```python
from build123d import *

# Parameters (mm, degrees)
F2_R        = 42.2275
F0_DEPTH    = 11.1125
F3_T        = -3.175
F0_FACE_R   = 42.2275
F0_FACE_R_2 = 39.0525
F4_DEPTH    = 25.4


with BuildPart() as f0:
    # F2 (on Top) → F0 (new body)
    with BuildSketch(Plane.XY):
        Circle(F2_R)
    extrude(amount=-F0_DEPTH)

    # F3
    f3_openings = [f0.faces().sort_by_distance(p)[0] for p in [
        (0, 0, 0),
    ]]
    offset(amount=F3_T, openings=f3_openings)

    # F1 (on face) + F0_face (on face) → F4 (cut)
    with BuildSketch(Plane.XY.offset(-7.9375)):
        with BuildLine():
            ThreePointArc((-18.689399569, -34.29), (-39.0525, 0), (-18.689399569, 34.29))
            Line((-18.689399569, 34.29), (-44.45, 34.29))
            Line((-44.45, 34.29), (-44.45, -34.29))
            Line((-44.45, -34.29), (-18.689399569, -34.29))
        make_face()
        with BuildLine():
            ThreePointArc((-5.9242471252, -34.29), (-34.798, 0), (-5.9242471252, 34.29))
            Line((-5.9242471252, 34.29), (-18.689399569, 34.29))
            ThreePointArc((-18.689399569, 34.29), (-39.0525, 0), (-18.689399569, -34.29))
            Line((-18.689399569, -34.29), (-5.9242471252, -34.29))
        make_face()
        with BuildLine():
            Line((0, 34.29), (-5.9242471252, 34.29))
            ThreePointArc((-5.9242471252, 34.29), (-34.798, 0), (-5.9242471252, -34.29))
            Line((-5.9242471252, -34.29), (0, -34.29))
            ThreePointArc((0, -34.29), (-34.29, 0), (0, 34.29))
        make_face()
    with BuildSketch(Plane.XY):
        Circle(F0_FACE_R)
        Circle(F0_FACE_R_2, mode=Mode.SUBTRACT)
    extrude(amount=F4_DEPTH, mode=Mode.SUBTRACT)


solid = f0.part
```
CAD build for the part. Positions are in the model's coordinates, mm. A direction names the side the tool comes from. Coordinates: 2 decimals unless noted, no trailing zeros. Order: outer loops, then holes, each group sorted by start corner. A loop starts at its lowest first (then second) coordinate and runs counter-clockwise, first axis right, second up. Notation, with made-up numbers: (84.25, -25.5) - (116.25, -25.5) arc R23 cw to (116.25, -15.5) - close; hole circle Ø8 at (-31.5, 25.5). An arc over 180 degrees is marked (long way). Use a Markdown table: item, result. Add a question column.
(1) Saw through at C-C (z = -10). Give the cut face in (x, y) (1 decimal).
(2) Saw through at A-A (x = 0). Give the cut face in (y, z), then the cut area to 3 significant figures.
(3) Drill centre lines: line 1 along Y through (x, z) = (0, -3); line 2 along Z through (x, y) = (-22, -17.5); line 3 along Y through (x, z) = (-24, -4.5). Where is each one in solid material? Low to high. Write a range as [from, to].
(4) Saw through at D-D (x = 24). Give the cut face in (y, z), then the cut area to 3 significant figures.
(5) Pull direction Y, two halves, no side cores. Call faces 1 (the face through (39.036, -1.131, -3.913)), 2 (the face through (38, 10, 0)), 3 (the face through (39.01, -16.17, -5.48)): +Y half, -Y half, draft (parallel to the pull), parting line (faces both ways), or undercut.
(6) Flat gauge pins, fed straight in: pin 1 (6 mm diameter, centred on x = 18.5, z = -4, fed in from -Y); pin 2 (1.5 mm diameter, centred on y = -13.5, z = -9.5, fed in from +X); pin 3 (8 mm diameter, centred on x = 16, y = -8, fed in from +Z). Where does each tip first touch, or does it go through?
(7) Saw through at B-B (y = 0). Give the cut face in (x, z).
(8) Which spindle directions (+Z, -Z, +X, -X, +Y, -Y) get a long thin tool onto all of the face, cutting with end or side? Do faces 4 (the face through (-1, 1, -11.112)), 5 (the face through (-22, -34.29, -4)). Say none if no direction does.
Solved:
| question | item | result |
|---|---|---|
| 1 | outline | circle Ø84.5 at (0, 0) |
| 2 | outline | (-42.23, -11.11) - (42.23, -11.11) - (42.23, 0) - (39.05, 0) - (39.05, -7.94) - (-39.05, -7.94) - (-39.05, 0) - (-42.23, 0) - close |
| 2 | area | 319 mm² |
| 3 | line 1 | y = [-42.23, -39.05], [39.05, 42.23] |
| 3 | line 2 | z = [-11.11, -7.94] |
| 3 | line 3 | y = [-34.74, -34.29], [34.29, 34.74] |
| 4 | outline | (-34.74, -11.11) - (34.74, -11.11) - (34.74, 0) - (30.81, 0) - (30.81, -7.94) - (-30.81, -7.94) - (-30.81, 0) - (-34.74, 0) - close |
| 4 | area | 283 mm² |
| 5 | face 1 | undercut |
| 5 | face 2 | draft |
| 5 | face 3 | parting line |
| 6 | pin 1 | stops at y = -39.28 |
| 6 | pin 2 | stops at x = 40.26 |
| 6 | pin 3 | stops at z = -7.94 |
| 7 | outline | (-42.23, -11.11) - (42.23, -11.11) - (42.23, 0) - (39.05, 0) - (39.05, -7.94) - (-42.23, -7.94) - close |
| 8 | face 4 | -Z, +X, -X, +Y, -Y |
| 8 | face 5 | +Z, -X |
